Can you work these out from the model? Positions are in its coordinate system, mm. A direction names the side the tool comes from. Give positions to 0.01 mm unless a question says otherwise; leave off trailing zeros. Write each loop counter-clockwise with the first axis right and the second up, starting at its lowest first coordinate (ties: lowest second). Pieces come first, ordered by that corner, then holes.
```python
from build123d import *

# Parameters (mm, degrees)
SKETCH1_W               = 8
SKETCH1_H               = 8
BOSS_EXTRUDE1_DEPTH     = 3
CUT_EXTRUDE1_DEPTH      = 12.704699911
CUT_EXTRUDE1_DEPTH_BACK = 12.704699911
CUT_EXTRUDE2_DEPTH      = 11
SKETCH4_R               = 1.8
CUT_EXTRUDE3_DEPTH      = 0.8
SKETCH5_W               = 8
SKETCH5_H               = 1
BOSS_EXTRUDE2_DEPTH     = 2
FILLET1_R               = 4
CUT_EXTRUDE4_DEPTH      = 0.4


with BuildPart() as part:
    # Sketch1 → Boss-Extrude1 (new body)
    with BuildSketch(Plane(origin=(0, 0, 0), x_dir=(1, 0, 0), z_dir=(0, 1, 0))):
        with Locations((4, 4)):
            Rectangle(SKETCH1_W, SKETCH1_H)
    extrude(amount=BOSS_EXTRUDE1_DEPTH)

    # Sketch2 → Cut-Extrude1 (cut, two sides: drawn at the far end of the back side and taken through both)
    with BuildSketch(Plane.XY.offset(-CUT_EXTRUDE1_DEPTH_BACK)):
        Polygon((0, 0), (0.6, 3), (0, 3), align=None)
        Polygon((8, 0), (7.4, 3), (8, 3), align=None)
    extrude(amount=CUT_EXTRUDE1_DEPTH + CUT_EXTRUDE1_DEPTH_BACK, mode=Mode.SUBTRACT)

    # Sketch3 → Cut-Extrude2 (cut)
    with BuildSketch(Plane(origin=(0, 0, 0), x_dir=(0, 0, -1), z_dir=(1, 0, 0))):
        Polygon((0, 0), (0.6, 3), (0, 3), align=None)
        Polygon((8, 3), (7.4, 3), (8, 0), align=None)
    extrude(amount=CUT_EXTRUDE2_DEPTH, mode=Mode.SUBTRACT)

    # Sketch4 → Cut-Extrude3 (cut)
    with BuildSketch(Plane.XZ):
        with Locations(Location((4, -3.75, 0), (0, 0, 270))):
            Circle(SKETCH4_R)
    extrude(amount=-CUT_EXTRUDE3_DEPTH, mode=Mode.SUBTRACT)

    # Sketch5 → Boss-Extrude2 (add)
    with BuildSketch(Plane.XZ):
        with Locations((4, -7.5)):
            Rectangle(SKETCH5_W, SKETCH5_H)
    extrude(amount=BOSS_EXTRUDE2_DEPTH)

    # Fillet1
    # the kernel refuses this fillet: 4 mm, written as the material it takes off along each edge
    with BuildSketch(Plane(origin=(8, -2, -16.660254038), x_dir=(0, 1, 0), z_dir=(0, 0, 1)), Plane(origin=(0, -2, 1.660254038), x_dir=(0, 1, 0), z_dir=(0, 0, -1))) as fillet1_piece_1:
        with BuildLine():
            CenterArc((4, 3.464101615), FILLET1_R, 180, 60)
            Line((0, 3.464101615), (-0.08, 3.464101615))
            Line((-0.08, 3.464101615), (-0.08, 0))
            Line((-0.08, 0), (0, -0.08))
            ThreePointArc((0, -0.08), (1, -0.08), (1.96, -0.069282032))
            Line((1.96, -0.069282032), (2, 0))
        make_face()
    extrude(amount=18.320508076, mode=Mode.SUBTRACT)

    # Sketch6 → Cut-Extrude4 (cut)
    with BuildSketch(Plane(origin=(0, 3, 0), x_dir=(1, 0, 0), z_dir=(0, 1, 0))):
        Polygon((3.605424489, 1.979723732), (2.126257822, 5.979723732), (2.938757822, 5.979723732), (3.998052694, 3.005364758), (5.053341155, 5.979723732), (5.869847566, 5.979723732), (4.396289873, 1.979723732), align=None)
    extrude(amount=-CUT_EXTRUDE4_DEPTH, mode=Mode.SUBTRACT)


solid = part.part
```
1) Suppose I cut it at D-D on x = 3.25. Write out the boundary of the cut face in (y, z), plus the area to 3 significant figures.
Values follow:
outline: (-1.99, -8) - (0, -8) - (3, -7.4) - (3, -5.11) - (2.6, -5.11) - (2.6, -2.94) - (3, -2.94) - (3, -0.6) - (0, 0) - (0, -2.11) - (0.8, -2.11) - (0.8, -5.39) - (0, -5.39) - (0, -7) - (-1.99, -7) - close
area: 20.7 mm2
2) For pin 1 Ø3 at (x, z) = (5, -4.5) entering from -Y, with a flat end and sliding along its axis, tell me the tip position at first contact or that it passes through.
Values follow:
pin 1: stops at y = 0
3) For faces 4 (the face through (4.541, 0.394, -5.467)), 5 (the face through (2.876, 2.803, -3.952)), 6 (the face through (1.49, -1.48, -7.49)), 7 (the face through (4, -1, -7)), which set-ups out of +Z, -Z, +X, -X, +Y, -Y let a thin tool reach every point of the face, with its end or its side?
Values follow:
face 4: -Y
face 5: +Y
face 6: +Z, -Z, -X, -Y
face 7: +Z, +X, -X, -Y
4) If we mould it in two halves opening along Z, with no side actions, what happens to faces 1 (the face through (3.9, 1.5, -0.3)), 2 (the face through (5.143, 2.803, -4.008)), 3 (the face through (3, 0, -2))? For each: +Z half, -Z half, draft (parallel to the pull), parting line (faces both ways), or undercut.
Values follow:
face 1: +Z half
face 2: undercut
face 3: draft
5) Please list where these lines run through material, in increasing order: L1, parallel to Z at x = 6.5, y = -0.7; L2, parallel to Y at x = 7.25, z = -6; L3, parallel to X at y = 0.6, z = -3.75.
Values follow:
L1: z = -8 to -7
L2: y = 0 to 3
L3: x = 0.12 to 2.2, 5.8 to 7.88
6) Suppose I cut it at B-B on z = -4. Write out the boundary of the cut face in (x, y).
Values follow:
outline: (0, 0) - (2.22, 0) - (2.22, 0.8) - (5.78, 0.8) - (5.78, 0) - (8, 0) - (7.4, 3) - (5.14, 3) - (5.14, 2.6) - (4.35, 2.6) - (4.35, 3) - (3.64, 3) - (3.64, 2.6) - (2.86, 2.6) - (2.86, 3) - (0.6, 3) - close
7) Suppose I cut it at A-A on x = 5.5. Write out the boundary of the cut face in (y, z), plus the area to 3 significant figures.
Values follow:
outline: (-1.88, -8) - (0, -8) - (3, -7.4) - (3, -5.98) - (2.6, -5.98) - (2.6, -4.98) - (3, -4.98) - (3, -0.6) - (0, 0) - (0, -2.76) - (0.8, -2.76) - (0.8, -4.74) - (0, -4.74) - (0, -7) - (-1.88, -7) - close
area: 22.1 mm2
8) Suppose I cut it at C-C on y = 2.2. Write out the boundary of the cut face in (x, z), plus the area to 3 significant figures.
Values follow:
outline: (0.44, -7.56) - (7.56, -7.56) - (7.56, -0.44) - (0.44, -0.44) - close
area: 50.7 mm2
